Input: part model. Units: mm. Frame: model coordinates. A direction names the side the tool comes from. Round coordinates to 2 decimals unless told otherwise and drop trailing zeros. Loops run counter-clockwise (first coordinate to the right, second up) from the corner with the lowest first, then second, coordinate; pieces in that order, holes last. Notation, with made-up numbers: (89, 44.25) -> (93, 44.25) arc R13 ccw to (93, 53.25) -> close; hole circle Ø3 at (70, 37). An arc over 180 degrees is marked (long way). Answer as a JSON object with one key per item and string values. Group by question number.
Item 1: Section query A-A on z = 0. Return loops of the section in (x, y).
Item 2: Set-up query: faces 4 (the flat face through (0, -5.3, -5.3)), 5 (the flat face through (-5, -2, 3)). Return all of +Z, -Z, +X, -X, +Y, -Y with unobstructed straight access to the full face (end or side cutting, diameter ignored); none if empty.
Item 3: Section query B-B on y = 0. Return loops of the section in (x, z).
Item 4: Section query C-C on x = -2.5. Return loops of the section in (y, z).
Item 5: Material intervals for line 1 (X direction, y = -5, z = 0); line 2 (X direction, y = 9.5, z = -18.5); line 3 (Z direction, x = -2.5, y = -4.6), sorted ascending. Write a range as [from, to].
Item 6: Draft query along Y for faces 1 (the cylindrical face through (-2.44, -1.15, 2.77)), 2 (the flat face through (0.2, -5, 0)), 3 (the cylindrical face through (-2.46, -6.43, 3.35)). Return one class per face: released by +Y, released by -Y, zero draft, split by the parting line, or undercut.
Item 7: Section query D-D on z = 6. Return loops of the section in (x, y).
Item 8: Pin query (flat end, axial travel): pin 1 (3 mm diameter, centred on x = -2.5, z = 0, fed in from +Y); pin 2 (6 mm diameter, centred on y = 13, z = -15, fed in from -X); pin 3 (1.5 mm diameter, centred on x = -2.5, z = 0, fed in from +Y); pin 4 (1.5 mm diameter, centred on x = -1.5, y = -4, fed in from +Z). Return the tip coordinate at first contact, or that it passes through.
from build123d import *

# Parameters (mm, degrees)
SKETCH_1_R                      = 25.25
EXTRUDE_1_DEPTH                 = 0.2
SKETCH_2_R                      = 7.25
EXTRUDE_2_DEPTH                 = 5
CUT_EXTRUDE_1_REACH             = 38.086
SKETCH_3_R                      = 3
CUT_EXTRUDE_2_REACH             = 38.057
SKETCH_4_R                      = 1.25
CUT_EXTRUDE_2_DIRECTION_2_REACH = 38.057


with BuildPart() as part:
    # 草图1 → 凸台-拉伸1 (new body)
    with BuildSketch(Plane(origin=(0, 0, 0), x_dir=(0, 0, -1), z_dir=(1, 0, 0))):
        Circle(SKETCH_1_R)
    extrude(amount=EXTRUDE_1_DEPTH)

    # 草图2 → 凸台-拉伸2 (add)
    with BuildSketch(Plane.ZY):
        Circle(SKETCH_2_R)
    extrude(amount=EXTRUDE_2_DEPTH)

    # 草图3 → 切除-拉伸1 (cut, up to next)
    with BuildSketch(Plane.ZY.offset(5), mode=Mode.PRIVATE) as cut_extrude_1_sk1:
        Circle(SKETCH_3_R)
    cut_extrude_1_tool1 = extrude(cut_extrude_1_sk1.sketch, amount=-CUT_EXTRUDE_1_REACH, mode=Mode.PRIVATE) & part.part
    add(cut_extrude_1_tool1.solids().sort_by_distance((-5, 0, 0))[0], mode=Mode.SUBTRACT)

    # 草图4 → 切除-拉伸2 (cut, up to next)
    with BuildSketch(Plane(origin=(0, 0, 0), x_dir=(1, 0, 0), z_dir=(0, 1, 0)), mode=Mode.PRIVATE) as cut_extrude_2_sk1:
        with Locations(Location((-2.5, 0, 0), (0, 0, 270))):
            Circle(SKETCH_4_R)
    cut_extrude_2_tool1 = extrude(cut_extrude_2_sk1.sketch, amount=-CUT_EXTRUDE_2_REACH, mode=Mode.PRIVATE) & part.part
    add(cut_extrude_2_tool1.solids().sort_by_distance((-2.5, 0, 0))[0], mode=Mode.SUBTRACT)

    # 草图4 → 切除-拉伸2 direction 2 (cut, up to next)
    with BuildSketch(Plane(origin=(0, 0, 0), x_dir=(1, 0, 0), z_dir=(0, 1, 0)), mode=Mode.PRIVATE) as cut_extrude_2_direction_2_sk1:
        with Locations(Location((-2.5, 0, 0), (0, 0, 270))):
            Circle(SKETCH_4_R)
    cut_extrude_2_direction_2_tool1 = extrude(cut_extrude_2_direction_2_sk1.sketch, amount=CUT_EXTRUDE_2_DIRECTION_2_REACH, mode=Mode.PRIVATE) & part.part
    add(cut_extrude_2_direction_2_tool1.solids().sort_by_distance((-2.5, 0, 0))[0], mode=Mode.SUBTRACT)


solid = part.part
Solved:
{
 "1": {"outline": "(-5, -7.25) -> (-3.75, -7.25) -> (-3.75, -3) -> (-5, -3) -> close; (-5, 3) -> (-3.75, 3) -> (-3.75, 7.25) -> (-5, 7.25) -> close; (-1.25, -7.25) -> (0, -7.25) -> (0, -25.25) -> (0.2, -25.25) -> (0.2, -3) -> (-1.25, -3) -> close; (-1.25, 3) -> (0.2, 3) -> (0.2, 25.25) -> (0, 25.25) -> (0, 7.25) -> (-1.25, 7.25) -> close"},
 "2": {"face 4": "-X", "face 5": "+Z, -Z, -X, +Y, -Y"},
 "3": {"outline": "(-5, -7.25) -> (0, -7.25) -> (0, -25.25) -> (0.2, -25.25) -> (0.2, -3) -> (-5, -3) -> close; (-5, 3) -> (0.2, 3) -> (0.2, 25.25) -> (0, 25.25) -> (0, 7.25) -> (-5, 7.25) -> close"},
 "4": {"outline": "(-7.14, -1.25) arc R7.25 ccw to (7.14, -1.25) -> (2.73, -1.25) arc R3 cw to (-2.73, -1.25) -> close; (-7.14, 1.25) -> (-2.73, 1.25) arc R3 cw to (2.73, 1.25) -> (7.14, 1.25) arc R7.25 ccw to start"},
 "5": {"line 1": "[-5, -3.75], [-1.25, 0.2]", "line 2": "[0, 0.2]", "line 3": "[-5.6, -1.25], [1.25, 5.6]"},
 "6": {"face 1": "undercut", "face 2": "zero draft", "face 3": "split by the parting line"},
 "7": {"outline": "(-5, -4.07) -> (0, -4.07) -> (0, -24.53) -> (0.2, -24.53) -> (0.2, 24.53) -> (0, 24.53) -> (0, 4.07) -> (-5, 4.07) -> close"},
 "8": {"pin 1": "y = 7.25", "pin 2": "x = 0", "pin 3": "through", "pin 4": "z = 6.48"}
}
